Check sheet for the modelled part. Datum: model origin and axes. Units: mm. A direction names the side the tool comes from. Round coordinates to 2 decimals unless told otherwise and drop trailing zeros. Write each loop counter-clockwise with the first axis right and the second up, starting at its lowest first coordinate (ties: lowest second). Pieces come first, ordered by that corner, then holes. Notation, with made-up numbers: (88, 67.5) -> (142, 67.5) arc R17 ccw to (142, 71.5) -> close; hole circle Ø5 at (13.5, -9.5). An arc over 180 degrees is marked (long way). One line per item, written item: value.
from build123d import *

# Parameters (mm, degrees)
BOSS_EXTRUDE1_DEPTH                          = 9.5
CBORE_FOR_M12_HEX_HEAD_CAP_SCREW2_AT_2_COUNT = 2
CBORE_FOR_M12_HEX_HEAD_CAP_SCREW2_AT_2_PITCH = 38.1


with BuildPart() as part:
    # Sketch1 → Boss-Extrude1 (new, symmetric)
    with BuildSketch(Plane(origin=(0, 0, 0), x_dir=(0, 0, -1), z_dir=(1, 0, 0))):
        with BuildLine():
            Line((25.4, 19), (-25.4, 19))
            Line((-25.4, 19), (-25.4, 0))
            Line((-25.4, 0), (-12.7, 0))
            ThreePointArc((-12.7, 0), (0, 12.7), (12.7, 0))
            Line((12.7, 0), (25.4, 0))
            Line((25.4, 0), (25.4, 19))
        make_face()
    extrude(amount=BOSS_EXTRUDE1_DEPTH, both=True)

    # Sketch8 → CBORE for M12 Hex Head Cap Screw2 (revolve, cut)
    with BuildSketch(Plane(origin=(0, 19, -19.05), x_dir=(0, 0, 1), z_dir=(1, 0, 0))):
        Polygon((0, 0), (0, 19), (6.775, 19), (3.375, 15.6), (3.375, 5), (12.5, 5), (12.5, 0), align=None)
    cbore_for_m12_hex_head_cap_screw2 = revolve(axis=Axis((0, 25.35, -19.05), (0, -1, 0)), mode=Mode.SUBTRACT)

    # CBORE for M12 Hex Head Cap Screw2 at 2: CBORE for M12 Hex Head Cap Screw2 ×2
    with Locations(*[(0, 0, i * CBORE_FOR_M12_HEX_HEAD_CAP_SCREW2_AT_2_PITCH) for i in range(1, CBORE_FOR_M12_HEX_HEAD_CAP_SCREW2_AT_2_COUNT)]):
        add(cbore_for_m12_hex_head_cap_screw2, mode=Mode.SUBTRACT)


solid = part.part
Item 1: Mould release check, pull along X, two halves, no side actions. Record for faces 4 (the flat face through (9.5, 14, 0)), 5 (the conical face through (1.356, 3.235, 22.32)), 6 (the flat face through (-9.5, 14, 0)): pulls with the +X half, pulls with the -X half, needs draft (parallel to the pull), parting line crosses it, or undercut.
Answer:
face 4: pulls with the +X half
face 5: undercut
face 6: pulls with the -X half
Item 2: Depth check by flat-ended pin: P1, Ø2, axis at x = -4.5, z = 9, coming from the +Y side; P2, Ø1, axis at x = 6, z = 20, coming from the -Y side; P3, Ø2, axis at x = 5.5, y = 15.5, coming from the +Z side; P4, Ø5.5, axis at x = 0, z = 19.05, coming from the -Y side. Enter the tip coordinate at first touch or a pass-through.
Answer:
P1: stops at y = 14
P2: stops at y = 0.2
P3: stops at z = 8.37
P4: passes through
Item 3: Sectioned sample at B-B on y = 10.75. Enter the section's corners in (x, z) (3 decimals), and give its area (3 significant figures).
Answer:
outline: (-9.5, -25.4) -> (9.5, -25.4) -> (9.5, -6.762) -> (-9.5, -6.762) -> close; (-9.5, 6.762) -> (9.5, 6.762) -> (9.5, 25.4) -> (-9.5, 25.4) -> close; hole circle Ø6.75 at (0, -19.05); hole circle Ø6.75 at (0, 19.05)
area: 637 mm^2
Item 4: Sectioned sample at D-D on y = 6.5. Enter the section's corners in (x, z) (3 decimals).
Answer:
outline: (-9.5, -25.4) -> (9.5, -25.4) -> (9.5, -10.911) -> (-9.5, -10.911) -> close; (-9.5, 10.911) -> (9.5, 10.911) -> (9.5, 25.4) -> (-9.5, 25.4) -> close; hole circle Ø6.75 at (0, -19.05); hole circle Ø6.75 at (0, 19.05)
Item 5: Tool access check on faces 1 (the flat face through (-7, 0, -19)), 2 (the cylindrical face through (0.15, 16.54, -6.55)), 3 (the cylindrical face through (-0.15, 16.54, 6.55)). Record the directions out of +Z, -Z, +X, -X, +Y, -Y that give a thin tool (end or side, any length) a straight path to the whole face; none if there is none.
Answer:
face 1: +Z, -Z, +X, -X, -Y
face 2: -Z, +Y
face 3: +Z, +Y
Item 6: Thickness scan on line 1 (X direction, y = 10, z = -19.05) (3 decimals); line 2 (Z direction, x = -2, y = 9.75); line 3 (Z direction, x = 0, y = 7.75) (3 decimals). Record the ranges inside material, lowest first.
Answer:
line 1: x = -9.5 to -3.375, 3.375 to 9.5
line 2: z = -25.4 to -21.77, -16.33 to -8.14, 8.14 to 16.33, 21.77 to 25.4
line 3: z = -25.4 to -22.425, -15.675 to -10.061, 10.061 to 15.675, 22.425 to 25.4
Item 7: Sectioned sample at C-C on x = 0. Enter the section's corners in (y, z) (3 decimals), and give its area (3 significant figures).
Answer:
outline: (0.418, -12.693) -> (3.4, -15.675) -> (14, -15.675) -> (14, -6.55) -> (19, -6.55) -> (19, 6.55) -> (14, 6.55) -> (14, 15.675) -> (3.4, 15.675) -> (0.418, 12.693) arc R12.7 cw to start; (0.425, -25.4) -> (14, -25.4) -> (14, -22.425) -> (3.4, -22.425) -> close; (0.425, 25.4) -> (3.4, 22.425) -> (14, 22.425) -> (14, 25.4) -> close
area: 312 mm^2
Item 8: Sectioned sample at A-A on z = 19.05. Enter the section's corners in (x, y) (3 decimals), and give its area (3 significant figures).
Answer:
outline: (-9.5, 0) -> (-6.775, 0) -> (-3.375, 3.4) -> (-3.375, 14) -> (-9.5, 14) -> close; (3.375, 3.4) -> (6.775, 0) -> (9.5, 0) -> (9.5, 14) -> (3.375, 14) -> close
area: 160 mm^2
